Could you check a few things on this model? Use its own coordinates, in mm. A direction names the side the tool comes from. Give positions to 0.01 mm unless a question says otherwise; leave off trailing zeros. Write each loop counter-clockwise with the first axis right and the second up, starting at its lowest first coordinate (ties: lowest second). Pieces come first, ordered by that corner, then holes. Notation, with made-up numbers: M 16.25,11 L 31.25,11 A34 cw 31.25,43 Z; hole C 84.5,38.25 d4. An arc over 180 degrees is marked long. Use one line per item in the form item = value.
from build123d import *

# Parameters (mm, degrees)
SKETCH_1_W          = 80
SKETCH_1_H          = 35.7
EXTRUDE_1_DEPTH     = 16
SHELL_1_T           = -2
CUT_EXTRUDE_3_REACH = 89.586
SKETCH_2_W          = 4.8
SKETCH_2_H          = 13.2
CUT_EXTRUDE_4_REACH = 89.586
SKETCH_6_R          = 2.5
SKETCH_6_W          = 3.16
SKETCH_6_H          = 8.94


with BuildPart() as part:
    # 草图1 → 凸台-拉伸1 (new body)
    with BuildSketch(Plane.XY):
        with Locations((-50.420566467, -11.517328482)):
            Rectangle(SKETCH_1_W, SKETCH_1_H)
        with BuildLine():
            Line((-10.420566467, -29.367328482), (-90.420566467, -29.367328482))
            ThreePointArc((-90.420566467, -29.367328482), (-50.420566467, -31.863413079), (-10.420566467, -29.367328482))
        make_face()
    extrude(amount=EXTRUDE_1_DEPTH)

    # 抽壳1
    shell_1_openings = [part.faces().sort_by_distance(p)[0] for p in [
        (-50.420566467, -12.357406874, 16),
        (-50.420566467, 6.332671518, 8),
        (-50.420566467, -31.863413079, 8),
    ]]
    offset(amount=SHELL_1_T, openings=shell_1_openings, kind=Kind.INTERSECTION)

    # 草图2 → 切除-拉伸3 (cut, up to next)
    with BuildSketch(Plane.ZY.offset(90.420566467), mode=Mode.PRIVATE) as cut_extrude_3_sk1:
        with Locations((8.4, -9.267328482)):
            Rectangle(SKETCH_2_W, SKETCH_2_H)
    cut_extrude_3_tool1 = extrude(cut_extrude_3_sk1.sketch, amount=-CUT_EXTRUDE_3_REACH, mode=Mode.PRIVATE) & part.part
    add(cut_extrude_3_tool1.solids().sort_by_distance((-90.420566, -9.267328, 8.4))[0], mode=Mode.SUBTRACT)

    # 草图6 → 切除-拉伸4 (cut, up to next)
    with BuildSketch(Plane(origin=(-10.420566467, 0, 0), x_dir=(0, 0, -1), z_dir=(1, 0, 0)), mode=Mode.PRIVATE) as cut_extrude_4_sk1:
        with Locations((-7.5, -10.607328482)):
            Circle(SKETCH_6_R)
    cut_extrude_4_tool1 = extrude(cut_extrude_4_sk1.sketch, amount=-CUT_EXTRUDE_4_REACH, mode=Mode.PRIVATE) & part.part
    # 草图6 → 切除-拉伸4 (cut, up to next)
    with BuildSketch(Plane(origin=(-10.420566467, 0, 0), x_dir=(0, 0, -1), z_dir=(1, 0, 0)), mode=Mode.PRIVATE) as cut_extrude_4_sk2:
        with Locations((-7.5, -17.607328482)):
            Circle(SKETCH_6_R)
    cut_extrude_4_tool2 = extrude(cut_extrude_4_sk2.sketch, amount=-CUT_EXTRUDE_4_REACH, mode=Mode.PRIVATE) & part.part
    # 草图6 → 切除-拉伸4 (cut, up to next)
    with BuildSketch(Plane(origin=(-10.420566467, 0, 0), x_dir=(0, 0, -1), z_dir=(1, 0, 0)), mode=Mode.PRIVATE) as cut_extrude_4_sk3:
        with Locations((-7.5, -24.607328482)):
            Circle(SKETCH_6_R)
    cut_extrude_4_tool3 = extrude(cut_extrude_4_sk3.sketch, amount=-CUT_EXTRUDE_4_REACH, mode=Mode.PRIVATE) & part.part
    # 草图6 → 切除-拉伸4 (cut, up to next)
    with BuildSketch(Plane(origin=(-10.420566467, 0, 0), x_dir=(0, 0, -1), z_dir=(1, 0, 0)), mode=Mode.PRIVATE) as cut_extrude_4_sk4:
        with Locations((-6.78, -1.137328482)):
            Rectangle(SKETCH_6_W, SKETCH_6_H)
    cut_extrude_4_tool4 = extrude(cut_extrude_4_sk4.sketch, amount=-CUT_EXTRUDE_4_REACH, mode=Mode.PRIVATE) & part.part
    add(cut_extrude_4_tool1.solids().sort_by_distance((-10.420566, -10.607328, 7.5))[0], mode=Mode.SUBTRACT)
    add(cut_extrude_4_tool2.solids().sort_by_distance((-10.420566, -17.607328, 7.5))[0], mode=Mode.SUBTRACT)
    add(cut_extrude_4_tool3.solids().sort_by_distance((-10.420566, -24.607328, 7.5))[0], mode=Mode.SUBTRACT)
    add(cut_extrude_4_tool4.solids().sort_by_distance((-10.420566, -1.137328, 6.78))[0], mode=Mode.SUBTRACT)


solid = part.part
1) If I drill on L1, parallel to X at y = 1.5, z = 12.5; L2, parallel to Y at x = -11.85, z = 7.5; L3, parallel to X at y = -18.5, z = 8.75, over which ranges is the centre line in solid material (lowest first)?
Checked values:
L1 = -90.42 to -88.42, -12.42 to -10.42
L2 = -29.54 to -27.11, -22.11 to -20.11, -15.11 to -13.11, -8.11 to -5.61, 3.33 to 6.33
L3 = -90.42 to -88.42
2) For faces 1 (the flat face through (-90.421, -12, 11)), 2 (the flat face through (-89, -9, 6)), 3 (the flat face through (-11, -5.607, 7)), 4 (the flat face through (-51, 6.333, 1)), 5 (the flat face through (-88.421, -12, 12)), which set-ups out of +Z, -Z, +X, -X, +Y, -Y let a thin tool reach every point of the face, with its end or its side?
Checked values:
face_1 = +Z, -Z, -X, +Y, -Y
face_2 = -X
face_3 = +X
face_4 = +Z, -Z, +X, -X, +Y
face_5 = +Z, +Y, -Y
3) I want a section at D-D, the plane z = 1.25. Please give me the cut outline in (x, y).
Checked values:
outline = M -90.42,-29.37 A321.75 ccw -10.42,-29.37 L -10.42,6.33 L -90.42,6.33 Z
4) I want a section at C-C, the plane z = 7.5. Please give me the cut outline in (x, y), plus the area to 3 significant figures.
Checked values:
outline = M -90.42,-29.37 A321.75 ccw -88.42,-29.61 L -88.42,-15.87 L -90.42,-15.87 Z; M -90.42,-2.67 L -88.42,-2.67 L -88.42,6.33 L -90.42,6.33 Z; M -12.42,-29.61 A321.75 ccw -10.42,-29.37 L -10.42,-27.11 L -12.42,-27.11 Z; M -12.42,-22.11 L -10.42,-22.11 L -10.42,-20.11 L -12.42,-20.11 Z; M -12.42,-15.11 L -10.42,-15.11 L -10.42,-13.11 L -12.42,-13.11 Z; M -12.42,-8.11 L -10.42,-8.11 L -10.42,-5.61 L -12.42,-5.61 Z; M -12.42,3.33 L -10.42,3.33 L -10.42,6.33 L -12.42,6.33 Z
area = 69.0 mm2
5) I want a section at B-B, the plane y = -21. Please give me the cut outline in (x, z), plus the area to 3 significant figures.
Checked values:
outline = M -90.42,0 L -10.42,0 L -10.42,16 L -12.42,16 L -12.42,2 L -88.42,2 L -88.42,16 L -90.42,16 Z
area = 216 mm2
6) For pin 1 Ø1.5 at (x, z) = (-41, 2) entering from -Y; pin 2 Ø2 at (x, z) = (-89.5, 9) entering from -Y; pin 3 Ø4 at (x, y) = (-60, -2) entering from +Z, each with a flat end and sliding along its axis, tell me the tip position at first contact or that it passes through.
Checked values:
pin_1 = -31.75
pin_2 = -29.6
pin_3 = 2
7) Thinking about a two-plate mould opening in Y: for faces 6 (the flat face through (-11, -11, 16)), 7 (the cylindrical face through (-50.608, -31.863, 1.444)), 8 (the flat face through (-89, -2.667, 8)), which applies, released by +Y, released by -Y, zero draft, split by the parting line, or undercut?
Checked values:
face_6 = zero draft
face_7 = released by -Y
face_8 = undercut
8) I want a section at A-A, the plane z = 11.75. Please give me the cut outline in (x, y).
Checked values:
outline = M -90.42,-29.37 A321.75 ccw -88.42,-29.61 L -88.42,6.33 L -90.42,6.33 Z; M -12.42,-29.61 A321.75 ccw -10.42,-29.37 L -10.42,6.33 L -12.42,6.33 Z
